from build123d import *

# Parameters (mm, degrees)
SKETCH_1_R      = 34.25
SKETCH_1_R_2    = 31.75
EXTRUDE_1_DEPTH = 150
SKETCH_3_R      = 34.25
EXTRUDE_2_DEPTH = 5
SKETCH_4_W      = 110
SKETCH_4_H      = 110
EXTRUDE_3_DEPTH = 3
SKETCH_5_W      = 110
SKETCH_5_H      = 110
SKETCH_5_W_2    = 105
SKETCH_5_H_2    = 105
EXTRUDE_4_DEPTH = 25


with BuildPart() as part:
    # 草圖1 → 填料-伸長1 (new body)
    with BuildSketch(Plane.XY):
        Circle(SKETCH_1_R)
        Circle(SKETCH_1_R_2, mode=Mode.SUBTRACT)
    extrude(amount=EXTRUDE_1_DEPTH)

    # 草圖3 → 填料-伸長2 (add)
    with BuildSketch(Plane.XY.offset(150)):
        Circle(SKETCH_3_R)
    extrude(amount=EXTRUDE_2_DEPTH)

    # 草圖4 → 填料-伸長3 (add)
    with BuildSketch(Plane.XY.offset(155)):
        with Locations((-55, 55)):
            Rectangle(SKETCH_4_W, SKETCH_4_H)
    extrude(amount=EXTRUDE_3_DEPTH)

    # 草圖5 → 填料-伸長4 (add)
    with BuildSketch(Plane.XY.offset(158)):
        with Locations((-55, 55)):
            Rectangle(SKETCH_5_W, SKETCH_5_H)
        with Locations((-55, 55)):
            Rectangle(SKETCH_5_W_2, SKETCH_5_H_2, mode=Mode.SUBTRACT)
    extrude(amount=EXTRUDE_4_DEPTH)


solid = part.part
Model file for the job. Use its own axes, mm. A direction names the side the tool comes from. Give positions to 0.01 mm unless a question says otherwise; leave off trailing zeros. Loops run counter-clockwise (first coordinate to the right, second up) from the corner with the lowest first, then second, coordinate; pieces in that order, holes last.
1) Saw through at D-D (y = 16). Write the cut outline in (x, z).
2) Pull direction Y, two halves, no side cores. Call faces 1 (the flat face through (0, 54, 169)), 2 (the flat face through (0, 0, 150)), 3 (the cylindrical face through (32.668, 10.288, 76.415)): +Y half, -Y half, draft (parallel to the pull), parting line (faces both ways), or undercut.
3) Flat gauge pins, fed straight in: pin 1 Ø8.5 at (y, z) = (69, 166) entering from +X; pin 2 Ø10 at (x, y) = (-80.5, 17) entering from +Z; pin 3 Ø19 at (x, y) = (6.5, -9) entering from -Z. Where does each tip first touch, or does it go through?
4) Saw through at A-A (x = -43). Write the cut outline in (y, z).
5) Tool access for faces 4 (the flat face through (-56, 0, 169)), 5 (the flat face through (-56, 2.5, 170)), 6 (the flat face through (-56, 56, 155)), 7 (the cylindrical face through (-6.883, -30.995, 73.95)): list every direction of +Z, -Z, +X, -X, +Y, -Y with a clear straight run to the whole face (end or side of a thin tool).
6) Saw through at C-C (z = 69.5). Write the cut outline in (x, y).
7) Wall check: line 1 (Y direction, x = 0, z = 90.5); line 2 (Z direction, x = -63, y = 6); line 3 (Z direction, x = 3, y = 27). Give the ranges that are in metal, low to high.
8) Saw through at B-B (y = 63). Write the cut outline in (x, z).
Answer block:
1. outline: (-110, 155) - (-30.28, 155) - (-30.28, 0) - (-27.42, 0) - (-27.42, 150) - (27.42, 150) - (27.42, 0) - (30.28, 0) - (30.28, 155) - (0, 155) - (0, 183) - (-2.5, 183) - (-2.5, 158) - (-107.5, 158) - (-107.5, 183) - (-110, 183) - close
2. face 1: draft
2. face 2: undercut
2. face 3: parting line
3. pin 1: stops at x = 0
3. pin 2: stops at z = 158
3. pin 3: stops at z = 150
4. outline: (0, 155) - (110, 155) - (110, 183) - (107.5, 183) - (107.5, 158) - (2.5, 158) - (2.5, 183) - (0, 183) - close
5. face 4: +Z, +X, -X, -Y
5. face 5: +Z
5. face 6: -Z, -X, +Y
5. face 7: -Z
6. outline: circle Ø68.5 at (0, 0); hole circle Ø63.5 at (0, 0)
7. line 1: y = -34.25 to -31.75, 31.75 to 34.25
7. line 2: z = 155 to 158
7. line 3: z = 150 to 155
8. outline: (-110, 155) - (0, 155) - (0, 183) - (-2.5, 183) - (-2.5, 158) - (-107.5, 158) - (-107.5, 183) - (-110, 183) - close
